from build123d import *

# Parameters (mm, degrees)
F0_R     = 27.25
F1_DEPTH = 8.6
F2_R     = 26.25
F3_DEPTH = 8
F4_R     = 25.25
F5_DEPTH = 7


with BuildPart() as f1:
    # F0 (on Top) → F1 (new body, symmetric)
    with BuildSketch(Plane.XY):
        Circle(F0_R)
    extrude(amount=F1_DEPTH, both=True)

    # F2 (on face) → F3 (cut)
    with BuildSketch(Plane.XY.offset(8.6)):
        Circle(F2_R)
    extrude(amount=-F3_DEPTH, mode=Mode.SUBTRACT)

    # F4 (on face) → F5 (cut)
    with BuildSketch(Plane(origin=(0, 0, -8.6), x_dir=(1, 0, 0), z_dir=(0, 0, -1))):
        Circle(F4_R)
    extrude(amount=-F5_DEPTH, mode=Mode.SUBTRACT)


solid = f1.part
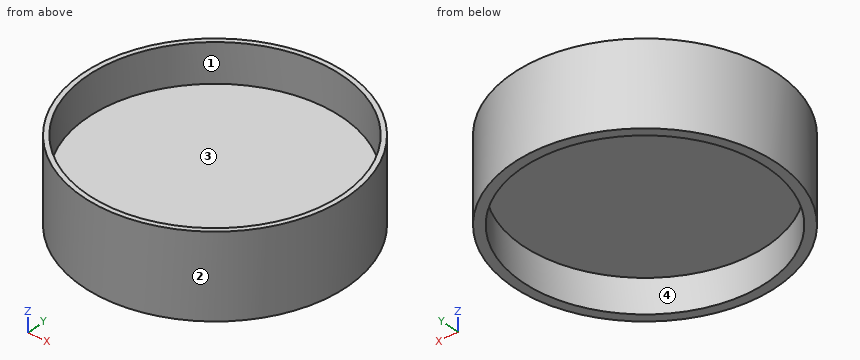
Read the model definition and answer for the solid it produces. Units are mm, in the model's axes. Face numbers are marked on the shaded views. A direction names the side the tool comes from. Round coordinates to 2 decimals unless told otherwise and drop trailing zeros. Write each loop counter-clockwise with the first axis right and the second up, starting at its lowest first coordinate (ties: lowest second). Pieces come first, ordered by that corner, then holes. Notation, with made-up numbers: M -24.75,27 L 33.25,27 A18 cw 33.25,44 Z; hole C 48,84.25 d3. An arc over 180 degrees is marked long. Use a Markdown table: item, result.
1) A tool of negligible diameter and unlimited length cuts with its end or side. For the marked faces 3 and 4, from which of +Z, -Z, +X, -X, +Y, -Y can it reach the whole face along a straight path? Write none if from no direction.
Answers follow:
| item | result |
|---|---|
| face 3 | +Z |
| face 4 | -Z |
2) The part is cut by section C-C (z = 1.5). Write down the section's boundary in (x, y).
Answers follow:
| item | result |
|---|---|
| outline | C 0,0 d54.5; hole C 0,0 d52.5 |
3) The part is cut by section D-D (z = -3.5). Write down the section's boundary in (x, y).
Answers follow:
| item | result |
|---|---|
| outline | C 0,0 d54.5; hole C 0,0 d50.5 |
4) Straight lines are drawn through the part: line 1 along Y through (x, z) = (0, 6); line 2 along Y through (x, z) = (0, -3.25); line 3 along X through (y, z) = (19, -3.5). For each, find the intervals that lie inside material, in ascending order. Write a range as [from, to].
Answers follow:
| item | result |
|---|---|
| line 1 | y = [-27.25, -26.25], [26.25, 27.25] |
| line 2 | y = [-27.25, -25.25], [25.25, 27.25] |
| line 3 | x = [-19.53, -16.63], [16.63, 19.53] |
5) The part is cut by section A-A (x = 0). Write down the section's boundary in (y, z).
Answers follow:
| item | result |
|---|---|
| outline | M -27.25,-8.6 L -25.25,-8.6 L -25.25,-1.6 L 25.25,-1.6 L 25.25,-8.6 L 27.25,-8.6 L 27.25,8.6 L 26.25,8.6 L 26.25,0.6 L -26.25,0.6 L -26.25,8.6 L -27.25,8.6 Z |
6) For a pull along Y with two mould halves and no side action, classify the marked faces 1 and 2 as pulls with the +Y half, pulls with the -Y half, needs draft (parallel to the pull), parting line crosses it, or undercut.
Answers follow:
| item | result |
|---|---|
| face 1 | undercut |
| face 2 | parting line crosses it |
7) Flat-ended cylindrical pins translate along their axes: pin 1 (3 mm diameter, centred on x = -19.5, z = -1, fed in from +Y); pin 2 (2 mm diameter, centred on x = -20.5, z = -0.5, fed in from +Y); pin 3 (5 mm diameter, centred on x = -16, z = 3.5, fed in from -Y). Find the tip coordinate at first contact, or state that the pin passes through.
Answers follow:
| item | result |
|---|---|
| pin 1 | stops at y = 20.46 |
| pin 2 | stops at y = 19.03 |
| pin 3 | stops at y = -23.67 |
